```python
from build123d import *

# Parameters (mm, degrees)
F0_W     = 10
F0_H     = 30
F0_W_2   = 8
F0_H_2   = 15
F0_R     = 17.5
F1_DEPTH = 15


with BuildPart() as f1:
    # F0 (on Top) → F1 (new body)
    with BuildSketch(Plane.XY):
        Polygon((-5.181603, 14.949999), (-160.181603, 14.949999), (-160.181603, -10.050001), (-150.181603, -10.050001), (-140.181603, -10.050001), (-132.181603, -10.050001), (-122.181603, -10.050001), (-112.181603, -10.050001), (-5.181603, -10.050001), align=None)
        with Locations((-155.181603, -25.050001)):
            Rectangle(F0_W, F0_H)
        with Locations((-136.181603, -17.550001)):
            Rectangle(F0_W_2, F0_H_2)
        Polygon((-117.290795, -25.050001), (-112.181603, -10.050001), (-122.181603, -10.050001), align=None)
        with BuildLine():
            ThreePointArc((-5.181603, -10.050001), (62.510139, 2.449999), (-5.181603, 14.949999))
            Line((-5.181603, 14.949999), (-5.181603, -10.050001))
        make_face()
        with Locations((27.510139, 2.449999)):
            Circle(F0_R, mode=Mode.SUBTRACT)
    extrude(amount=F1_DEPTH)


solid = f1.part
```
CAD build for the part. Positions are in the model's coordinates, mm. A direction names the side the tool comes from. Coordinates: 2 decimals unless noted, no trailing zeros. Write each loop counter-clockwise with the first axis right and the second up, starting at its lowest first coordinate (ties: lowest second). Pieces come first, ordered by that corner, then holes. Notation, with made-up numbers: (85.25, -31.75) -> (126.25, -31.75) arc R22 cw to (126.25, -1.75) -> close; hole circle Ø7 at (41, -9). An arc over 180 degrees is marked (long way). Return JSON: item names as keys, results as strings. Group by question number.
Q1. Flat gauge pins, fed straight in: pin 1 (8 mm diameter, centred on x = -145, z = 4, fed in from -Y); pin 2 (4.5 mm diameter, centred on y = -28.5, z = 10, fed in from +X); pin 3 (5 mm diameter, centred on x = -29, z = 7, fed in from +Y). Where does each tip first touch, or does it go through?
Q2. Which spindle directions (+Z, -Z, +X, -X, +Y, -Y) get a long thin tool onto all of the face, cutting with end or side? Do faces 1 (the face through (-136, -25.05, 7)), 2 (the face through (-26, -1, 0)). Say none if no direction does.
Q3. Cut at C-C, the plane y = -22. Give the cut face in (x, z).
Q4. Drill centre lines: line 1 (X direction, y = -24.5, z = 4.75); line 2 (Y direction, x = -36, z = 13); line 3 (X direction, y = 11.5, z = 13.5). Where is each one in solid material? Low to high.
Q5. Cut at D-D, the plane x = 28. Give the cut face in (y, z), then the cut area to 3 significant figures.
Q6. Pull direction X, two halves, no side cores. Call faces 3 (the face through (-82, 14.95, 7)), 4 (the face through (62.484, 1.09, 7.395)), 5 (the face through (-160.182, -12, 7)): released by +X, released by -X, zero draft, split by the parting line, or undercut.
Q7. Cut at B-B, the plane z = 13. Give the cut face in (x, y).
Q8. Cut at A-A, the plane y = -7.5. Give the cut face in (x, z).
Returned:
{
 "1": {"pin 1": "stops at y = -10.05", "pin 2": "stops at x = 47.54", "pin 3": "stops at y = 14.95"},
 "2": {"face 1": "+Z, -Z, -Y", "face 2": "-Z, +X, -X, +Y, -Y"},
 "3": {"outline": "(-160.18, 0) -> (-150.18, 0) -> (-150.18, 15) -> (-160.18, 15) -> close; (-140.18, 0) -> (-132.18, 0) -> (-132.18, 15) -> (-140.18, 15) -> close; (-118.29, 0) -> (-116.25, 0) -> (-116.25, 15) -> (-118.29, 15) -> close; (2.47, 0) -> (52.55, 0) -> (52.55, 15) -> (2.47, 15) -> close"},
 "4": {"line 1": "x = -160.18 to -150.18, -140.18 to -132.18, -117.47 to -117.1, 5.18 to 49.84", "line 2": "y = -10.05 to 14.95", "line 3": "x = -160.18 to 12.53, 42.49 to 61.32"},
 "5": {"outline": "(-32.55, 0) -> (-15.04, 0) -> (-15.04, 15) -> (-32.55, 15) -> close; (19.94, 0) -> (37.45, 0) -> (37.45, 15) -> (19.94, 15) -> close", "area": "525 mm2"},
 "6": {"face 3": "zero draft", "face 4": "undercut", "face 5": "released by -X"},
 "7": {"outline": "(-160.18, -40.05) -> (-150.18, -40.05) -> (-150.18, -10.05) -> (-140.18, -10.05) -> (-140.18, -25.05) -> (-132.18, -25.05) -> (-132.18, -10.05) -> (-122.18, -10.05) -> (-117.29, -25.05) -> (-112.18, -10.05) -> (-5.18, -10.05) arc R35 ccw (long way) to (-5.18, 14.95) -> (-160.18, 14.95) -> close; hole circle Ø35 at (27.51, 2.45)"},
 "8": {"outline": "(-160.18, 0) -> (13.11, 0) -> (13.11, 15) -> (-160.18, 15) -> close; (41.91, 0) -> (61.07, 0) -> (61.07, 15) -> (41.91, 15) -> close"}
}
